Verification items for the finished model (mm, model axes). Face numbers are marked on the shaded views. A direction names the side the tool comes from. Round coordinates to 2 decimals unless told otherwise and drop trailing zeros. Order: outer loops, then holes, each group sorted by start corner. A loop starts at its lowest first (then second) coordinate and runs counter-clockwise, first axis right, second up. Notation, with made-up numbers: (19.25, 76.25) -> (34.25, 76.25) arc R21 cw to (34.25, 80.25) -> close; hole circle Ø3 at (57, -2.75). An arc over 180 degrees is marked (long way). Return JSON: item names as keys, results as strings. Group by question number.
Item 1: Sectioned sample at B-B on y = 9. Record the cut outline in (x, z).
Item 2: Scan lines: probe 1 along X at (y, z) = (34, 7); probe 2 along Y at (x, z) = (61, 19); probe 3 along X at (y, z) = (8.5, 9). Record each from-to range of solid material in increasing order. Write a range as from..to.
Item 3: Draft check along X on the marked faces 1, 2 and 3. Enter one of: pulls with the +X half, pulls with the -X half, needs draft (parallel to the pull), parting line crosses it, or undercut.
Item 4: Sectioned sample at C-C on x = 37.5. Record the cut outline in (y, z), plus the area to 3 significant figures.
Item 5: Sectioned sample at A-A on x = -30. Record the cut outline in (y, z).
Item 6: Depth check by flat-ended pin: pin 1 Ø2 at (x, y) = (19, -24) entering from +Z; pin 2 Ø1.5 at (y, z) = (52.5, 24) entering from -X; pin 3 Ø1.5 at (y, z) = (51, 30.5) entering from -X. Enter the tip coordinate at first touch or a pass-through.
Item 7: Access from +Z, -Z, +X, -X, +Y, -Y to the whole of each face (thin tool, end or side, straight path). Record for the marked faces 4 and 5.
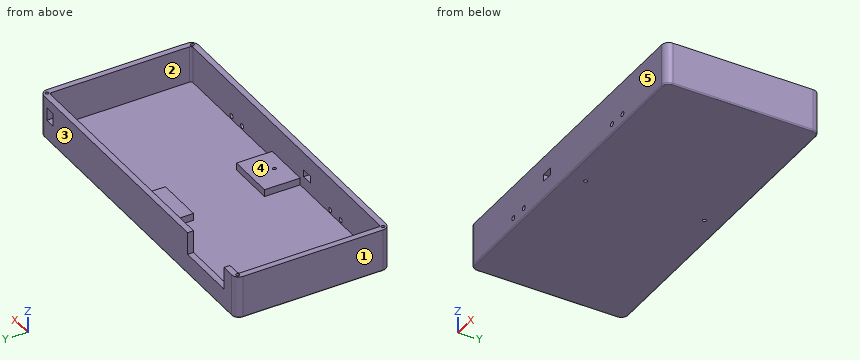
```python
from build123d import *

# Parameters (mm, degrees)
F0_W      = 280
F0_H      = 130
F1_DEPTH  = 36
F2_W      = 270
F2_H      = 120
F3_DEPTH  = 31
F4_R      = 2
F4_W      = 10
F4_H      = 6
F6_DEPTH  = 25
F5_W      = 52
F5_H      = 19
F5_W_2    = 9
F5_H_2    = 11
F7_DEPTH  = 25
F8_W      = 40
F8_H      = 30
F9_DEPTH  = 11
F10_R     = 1.5
F11_DEPTH = 12
F12_R     = 1.5
F13_DEPTH = 12
F14_R     = 6
F15_R     = 2
F16_R     = 1


# Not quite as in the source:
# - a feature names something its author has since deleted; it is built from what else it names


with BuildPart() as f1:
    # F0 (on Top) → F1 (new body)
    with BuildSketch(Plane.XY):
        with Locations((-12.5971958935, -11.2710741152)):
            Rectangle(F0_W, F0_H)
    extrude(amount=F1_DEPTH)

    # F2 (on face) → F3 (cut)
    with BuildSketch(Plane.XY.offset(36)):
        with Locations((-12.5971958935, -11.2710741152)):
            Rectangle(F2_W, F2_H)
    extrude(amount=-F3_DEPTH, mode=Mode.SUBTRACT)

    # F4 (on face) → F6 (cut)
    with BuildSketch(Plane.XZ.offset(76.2710741152)):
        with Locations((-90.5971958935, 8)):
            Circle(F4_R)
        with Locations((-75.5971958935, 8)):
            Circle(F4_R)
        with Locations((50.4028041065, 8)):
            Circle(F4_R)
        with Locations((65.4028041065, 8)):
            Circle(F4_R)
        with Locations((-42.5971958935, 18)):
            Rectangle(F4_W, F4_H)
    extrude(amount=-F6_DEPTH, mode=Mode.SUBTRACT)

    # F5 (on face) → F7 (cut)
    with BuildSketch(Plane(origin=(0, 53.7289258848, 0), x_dir=(-1, 0, 0), z_dir=(0, 1, 0))):
        with Locations((109.5971958935, 26.5)):
            Rectangle(F5_W, F5_H)
        with Locations((-112.9028041065, 22.5)):
            Rectangle(F5_W_2, F5_H_2)
    extrude(amount=-F7_DEPTH, mode=Mode.SUBTRACT)

    # F8 (on face) → F9 (join)
    with BuildSketch(Plane(origin=(0, 0, 0), x_dir=(1, 0, 0), z_dir=(0, 0, -1))):
        with Locations((-12.5971958935, -33.7289258848)):
            Rectangle(F8_W, F8_H)
        with Locations((-12.5971958935, 56.2710741152)):
            Rectangle(F8_W, F8_H)
    extrude(amount=-F9_DEPTH)

    # F10 (on face) → F11 (cut)
    with BuildSketch(Plane.XY.offset(11)):
        with Locations((-12.5971958935, 38.7289258848)):
            Circle(F10_R)
        with Locations((-12.5971958935, -61.2710741152)):
            Circle(F10_R)
    extrude(amount=-F11_DEPTH, mode=Mode.SUBTRACT)

    # F12 (on face) → F13 (cut)
    with BuildSketch(Plane.XY.offset(36)):
        with Locations((-148.8471958935, 49.9789258848)):
            Circle(F12_R)
        with Locations((-148.8471958935, -72.5210741152)):
            Circle(F12_R)
        with Locations((123.6528041065, -72.5210741152)):
            Circle(F12_R)
        with Locations((123.6528041065, 49.9789258848)):
            Circle(F12_R)
    extrude(amount=-F13_DEPTH, mode=Mode.SUBTRACT)

    # F14
    f14_edges = [f1.edges().sort_by_distance(p)[0] for p in [
        (-152.597196, -76.271074, 18),
        (-152.597196, 53.728926, 18),
        (127.402804, -76.271074, 18),
        (127.402804, 53.728926, 18),
    ]]
    fillet(f14_edges, radius=F14_R)

    # F15
    f15_edges = [f1.edges().sort_by_distance(p)[0] for p in [
        (-147.597196, 48.728926, 20.5),
        (-147.597196, -71.271074, 20.5),
        (122.402804, 48.728926, 20.5),
        (122.402804, -71.271074, 20.5),
    ]]
    fillet(f15_edges, radius=F15_R)

    # F16
    f16_edges = [f1.edges().sort_by_distance(p)[0] for p in [
        (-152.597196, -11.271074, 0),
    ]]
    fillet(f16_edges, radius=F16_R)


solid = f1.part
```
Recorded:
{
 "1": {"outline": "(-152.6, 1) arc R1 ccw to (-151.6, 0) -> (126.4, 0) arc R1 ccw to (127.4, 1) -> (127.4, 36) -> (122.4, 36) -> (122.4, 5) -> (-147.6, 5) -> (-147.6, 36) -> (-152.6, 36) -> close"},
 "2": {"probe 1": "-152.6..-147.6, -32.6..7.4, 122.4..127.4", "probe 2": "-76.27..-71.27, 48.73..53.73", "probe 3": "-152.6..-147.6, 122.4..127.4"},
 "3": {"face 1": "pulls with the -X half", "face 2": "undercut", "face 3": "needs draft"},
 "4": {"outline": "(-76.27, 1) arc R1 ccw to (-75.27, 0) -> (52.73, 0) arc R1 ccw to (53.73, 1) -> (53.73, 36) -> (48.73, 36) -> (48.73, 5) -> (-71.27, 5) -> (-71.27, 36) -> (-76.27, 36) -> close", "area": "960 mm²"},
 "5": {"outline": "(-76.27, 1) arc R1 ccw to (-75.27, 0) -> (52.73, 0) arc R1 ccw to (53.73, 1) -> (53.73, 36) -> (48.73, 36) -> (48.73, 11) -> (18.73, 11) -> (18.73, 5) -> (-41.27, 5) -> (-41.27, 11) -> (-71.27, 11) -> (-71.27, 36) -> (-76.27, 36) -> close"},
 "6": {"pin 1": "z = 5", "pin 2": "x = -151.05", "pin 3": "x = -152.04"},
 "7": {"face 4": "+Z", "face 5": "+Z, -Z, +X, -X, -Y"}
}
